from build123d import *

# Parameters (mm, degrees)
EXTRUDE_1_DEPTH     = 108.58
SKETCH_11_R         = 2
CUT_EXTRUDE_4_DEPTH = 3
SKETCH_12_R         = 1.3
CUT_EXTRUDE_5_DEPTH = 14
SKETCH_15_W         = 13
SKETCH_15_H         = 13
SKETCH_15_W_2       = 5
SKETCH_15_H_2       = 28
CUT_EXTRUDE_6_DEPTH = 10
CUT_EXTRUDE_7_DEPTH = 10
SKETCH_17_W         = 1.5
SKETCH_17_H         = 0.5299964
SKETCH_17_H_2       = 0.5300218
CUT_EXTRUDE_8_DEPTH = 3.813730334
SKETCH_18_W         = 5.08
SKETCH_18_H         = 2.54
EXTRUDE_2_DEPTH     = 7


with BuildPart() as part:
    # 草图3 → 凸台-拉伸1 (new body)
    with BuildSketch(Plane.XY):
        with BuildLine():
            Line((24.686269666, 24.686269666), (24.686269666, -24.686269666))
            ThreePointArc((24.686269666, -24.686269666), (30, 0), (24.686269666, 24.686269666))
        make_face()
    extrude(amount=EXTRUDE_1_DEPTH)

    # 草图11 → 切除-拉伸4 (cut)
    with BuildSketch(Plane(origin=(30, 0, 0), x_dir=(0, 0, -1), z_dir=(1, 0, 0))):
        with Locations((-1.254, -12.343134833)):
            Circle(SKETCH_11_R)
        with Locations((-1.254, 0)):
            Circle(SKETCH_11_R)
        with Locations((-1.254, 12.343134833)):
            Circle(SKETCH_11_R)
        with Locations((-107.33, -12.343134833)):
            Circle(SKETCH_11_R)
        with Locations((-107.33, 0)):
            Circle(SKETCH_11_R)
        with Locations((-107.33, 12.343134833)):
            Circle(SKETCH_11_R)
    extrude(amount=-CUT_EXTRUDE_4_DEPTH, mode=Mode.SUBTRACT)

    # 草图12 → 切除-拉伸5 (cut)
    with BuildSketch(Plane(origin=(27, 0, 0), x_dir=(0, 0, -1), z_dir=(1, 0, 0))):
        with Locations((-1.254, -12.343134833)):
            Circle(SKETCH_12_R)
        with Locations((-1.254, 0)):
            Circle(SKETCH_12_R)
        with Locations((-1.254, 12.343134833)):
            Circle(SKETCH_12_R)
        with Locations((-107.33, 12.343134833)):
            Circle(SKETCH_12_R)
        with Locations((-107.33, 0)):
            Circle(SKETCH_12_R)
        with Locations((-107.33, -12.343134833)):
            Circle(SKETCH_12_R)
    extrude(amount=-CUT_EXTRUDE_5_DEPTH, mode=Mode.SUBTRACT)

    # 草图15 → 切除-拉伸6 (cut)
    with BuildSketch(Plane.ZY.offset(-24.686269666)):
        with Locations((95.066746, -2.286)):
            Rectangle(SKETCH_15_W, SKETCH_15_H)
        with Locations((82.3670381, -3.555929665)):
            Rectangle(SKETCH_15_W_2, SKETCH_15_H_2)
        with Locations((73.5725421, -3.556070335)):
            Rectangle(SKETCH_15_W_2, SKETCH_15_H_2)
        with Locations((64.6825421, -3.555934352)):
            Rectangle(SKETCH_15_W_2, SKETCH_15_H_2)
        with Locations((55.7925421, -3.564457152)):
            Rectangle(SKETCH_15_W_2, SKETCH_15_H_2)
    extrude(amount=-CUT_EXTRUDE_6_DEPTH, mode=Mode.SUBTRACT)

    # 草图16 → 切除-拉伸7 (cut)
    with BuildSketch(Plane.ZY.offset(-24.686269666)):
        Polygon((100.135, -10.7730036), (100.135, -11.303), (101.925, -11.303), (101.925, -13.843), (100.135, -13.843), (100.135, -14.3730218), (102.4349812, -14.3730218), (102.4349812, -10.7730036), align=None)
        Polygon((96.3349934, -10.7730036), (96.3349934, -14.3730218), (98.635, -14.3730218), (98.635, -13.843), (96.845, -13.843), (96.845, -11.303), (98.635, -11.303), (98.635, -10.7730036), align=None)
        Polygon((102.4349812, -16.8690036), (100.135, -16.8690036), (100.135, -17.399), (101.925, -17.399), (101.925, -19.939), (100.135, -19.939), (100.135, -20.4690218), (102.4349812, -20.4690218), align=None)
        Polygon((96.3349934, -16.8690036), (96.3349934, -20.4690218), (98.635, -20.4690218), (98.635, -19.939), (96.845, -19.939), (96.845, -17.399), (98.635, -17.399), (98.635, -16.8690036), align=None)
        Polygon((93.7989812, -10.7730036), (91.499, -10.7730036), (91.499, -11.303), (93.289, -11.303), (93.289, -13.843), (91.499, -13.843), (91.499, -14.3730218), (93.7989812, -14.3730218), align=None)
        Polygon((87.6989934, -10.7730036), (87.6989934, -14.3730218), (89.999, -14.3730218), (89.999, -13.843), (88.209, -13.843), (88.209, -11.303), (89.999, -11.303), (89.999, -10.7730036), align=None)
        Polygon((93.7989812, -16.8690036), (91.499, -16.8690036), (91.499, -17.399), (93.289, -17.399), (93.289, -19.939), (91.499, -19.939), (91.499, -20.4690218), (93.7989812, -20.4690218), align=None)
        Polygon((87.6989934, -16.8690036), (87.6989934, -20.4690218), (89.999, -20.4690218), (89.999, -19.939), (88.209, -19.939), (88.209, -17.399), (89.999, -17.399), (89.999, -16.8690036), align=None)
    extrude(amount=-CUT_EXTRUDE_7_DEPTH, mode=Mode.SUBTRACT)

    # 草图17 → 切除-拉伸8 (cut)
    with BuildSketch(Plane(origin=(30, 0, 0), x_dir=(0, 0, -1), z_dir=(1, 0, 0))):
        with Locations((-99.385, -11.0380018)):
            Rectangle(SKETCH_17_W, SKETCH_17_H)
        with Locations((-99.385, -14.1080109)):
            Rectangle(SKETCH_17_W, SKETCH_17_H_2)
        with Locations((-99.385, -17.1340018)):
            Rectangle(SKETCH_17_W, SKETCH_17_H)
        with Locations((-99.385, -20.2040109)):
            Rectangle(SKETCH_17_W, SKETCH_17_H_2)
        with Locations((-90.749, -17.1340018)):
            Rectangle(SKETCH_17_W, SKETCH_17_H)
        with Locations((-90.749, -20.2040109)):
            Rectangle(SKETCH_17_W, SKETCH_17_H_2)
        with Locations((-90.749, -11.0380018)):
            Rectangle(SKETCH_17_W, SKETCH_17_H)
        with Locations((-90.749, -14.1080109)):
            Rectangle(SKETCH_17_W, SKETCH_17_H_2)
    extrude(amount=-CUT_EXTRUDE_8_DEPTH, mode=Mode.SUBTRACT)

    # 草图18 → 凸台-拉伸2 (add)
    with BuildSketch(Plane.ZY.offset(-24.686269666)):
        with Locations((90.749, -12.573)):
            Rectangle(SKETCH_18_W, SKETCH_18_H)
        with Locations((90.749, -18.669)):
            Rectangle(SKETCH_18_W, SKETCH_18_H)
        with Locations((99.385, -12.573)):
            Rectangle(SKETCH_18_W, SKETCH_18_H)
        with Locations((99.385, -18.669)):
            Rectangle(SKETCH_18_W, SKETCH_18_H)
    extrude(amount=EXTRUDE_2_DEPTH)


solid = part.part
Build history of the part. All positions in model axes, mm. A direction names the side the tool comes from. Coordinates: 2 decimals unless noted, no trailing zeros. Order: outer loops, then holes, each group sorted by start corner. A loop starts at its lowest first (then second) coordinate and runs counter-clockwise, first axis right, second up. Notation, with made-up numbers: (0.25, 82) -> (43.25, 82) arc R12 ccw to (43.25, 95) -> close; hole circle Ø9 at (-1, 36). An arc over 180 degrees is marked (long way). One line per item, written item: value.
(1) Tool access for faces 1 (the flat face through (27, -12, 3)), 2 (the flat face through (27, -4, 76.073)): list every direction of +Z, -Z, +X, -X, +Y, -Y with a clear straight run to the whole face (end or side of a thin tool).
Checked values:
face 1: +X
face 2: +X, -X
(2) Mould opens along Z. For faces 3 (the flat face through (23, -17.399, 91)), 4 (the cylindrical face through (27.832, -11.442, 105.545)), 5 (the flat face through (17.686, -19, 91)) say: pulls with the +Z half, pulls with the -Z half, needs draft (parallel to the pull), parting line crosses it, or undercut.
Checked values:
face 3: undercut
face 4: undercut
face 5: needs draft
(3) Probe line 1 (Z direction, x = 28.5, y = 7.5); line 2 (Z direction, x = 26.2, y = 0); line 3 (Y direction, x = 28.8, z = 107.33). List the from-to ranges inside material, lowest first. Write a range as [from, to].
Checked values:
line 1: [0, 53.29], [58.29, 62.18], [67.18, 71.07], [76.07, 79.87], [84.87, 108.58]
line 2: [2.55, 53.29], [58.29, 62.18], [67.18, 71.07], [76.07, 79.87], [84.87, 88.57], [101.57, 106.03]
line 3: [-10.34, -2], [2, 10.34]
(4) Slice it at D-D, the plane z = 47. List the corners of the cut face in (x, y), plus the area to 3 significant figures.
Checked values:
outline: (24.69, -24.69) arc R60 ccw to (24.69, 24.69) -> close
area: 177 mm2
(5) Slice it at C-C, the plane z = 64. List the corners of the cut face in (x, y).
Checked values:
outline: (24.69, -24.69) arc R60 ccw to (27.37, -17.56) -> (24.69, -17.56) -> close; (24.69, 10.44) -> (29.08, 10.44) arc R60 ccw to (24.69, 24.69) -> close
(6) Slice it at A-A, the plane x = 18.75. List the corners of the cut face in (y, z) (3 decimals), plus the area to 3 significant figures.
Checked values:
outline: (-19.939, 88.209) -> (-17.399, 88.209) -> (-17.399, 93.289) -> (-19.939, 93.289) -> close; (-19.939, 96.845) -> (-17.399, 96.845) -> (-17.399, 101.925) -> (-19.939, 101.925) -> close; (-13.843, 88.209) -> (-11.303, 88.209) -> (-11.303, 93.289) -> (-13.843, 93.289) -> close; (-13.843, 96.845) -> (-11.303, 96.845) -> (-11.303, 101.925) -> (-13.843, 101.925) -> close
area: 51.6 mm2
(7) Drop flat-ended pins along their axis: pin 1 Ø6 at (x, z) = (21, 46.5) entering from +Y; pin 2 Ø1.4 at (x, z) = (25.5, 91) entering from +Y; pin 3 Ø1.5 at (x, z) = (20.5, 91) entering from +Y; pin 4 Ø1.5 at (x, z) = (21.5, 99) entering from -Y. Give the stop position or say it passes through.
Checked values:
pin 1: through
pin 2: y = 24.43
pin 3: y = -11.3
pin 4: y = -19.94
(8) Slice it at B-B, the plane z = 107.33. List the corners of the cut face in (x, y).
Checked values:
outline: (24.69, -24.69) arc R60 ccw to (28.26, -14.34) -> (27, -14.34) -> (27, -13.64) -> (24.69, -13.64) -> close; (24.69, -11.04) -> (27, -11.04) -> (27, -10.34) -> (29.1, -10.34) arc R60 ccw to (29.97, -2) -> (27, -2) -> (27, -1.3) -> (24.69, -1.3) -> close; (24.69, 1.3) -> (27, 1.3) -> (27, 2) -> (29.97, 2) arc R60 ccw to (29.1, 10.34) -> (27, 10.34) -> (27, 11.04) -> (24.69, 11.04) -> close; (24.69, 13.64) -> (27, 13.64) -> (27, 14.34) -> (28.26, 14.34) arc R60 ccw to (24.69, 24.69) -> close
